```python
from build123d import *

# Parameters (mm, degrees)
BOSS_EXTRUDE1_DEPTH = 5
SKETCH2_R           = 4
CUT_EXTRUDE1_DEPTH  = 6


with BuildPart() as part:
    # Sketch1 → Boss-Extrude1 (new body)
    with BuildSketch(Plane(origin=(0, 0, 0), x_dir=(0, 0, -1), z_dir=(1, 0, 0))):
        with BuildLine():
            Line((-25, 10), (25, 10))
            ThreePointArc((25, 10), (35, 0), (25, -10))
            Line((25, -10), (-25, -10))
            ThreePointArc((-25, -10), (-35, 0), (-25, 10))
        make_face()
    extrude(amount=BOSS_EXTRUDE1_DEPTH)

    # Sketch2 → Cut-Extrude1 (cut, through all)
    with BuildSketch(Plane(origin=(5, 0, 0), x_dir=(0, 0, -1), z_dir=(1, 0, 0))):
        with Locations((-25, 0)):
            Circle(SKETCH2_R)
        with Locations((25, 0)):
            Circle(SKETCH2_R)
    extrude(amount=-CUT_EXTRUDE1_DEPTH, mode=Mode.SUBTRACT)


solid = part.part
```
Design review of the part built by this model. Coordinates are the model's own, in mm. Coordinates: 2 decimals unless noted, no trailing zeros. Loops run counter-clockwise (first coordinate to the right, second up) from the corner with the lowest first, then second, coordinate; pieces in that order, holes last.
Q1. We need section D-D on y = -3. State the section outline as (x, z) points, and give its area (3 significant figures).
Reported:
outline: (0, -34.54) - (5, -34.54) - (5, -27.65) - (0, -27.65) - close; (0, -22.35) - (5, -22.35) - (5, 22.35) - (0, 22.35) - close; (0, 27.65) - (5, 27.65) - (5, 34.54) - (0, 34.54) - close
area: 292 mm2
Q2. For pin 1 (9 mm diameter, centred on y = 0, z = -25, fed in from -X); pin 2 (3 mm diameter, centred on x = 1.5, y = -7.5, fed in from -Z); pin 3 (1 mm diameter, centred on x = 3, y = -7.5, fed in from +Z), all flat-tipped, find the tip position at first contact; note any pin that passes through.
Reported:
pin 1: stops at x = 0
pin 2: stops at z = -33
pin 3: stops at z = 32.14
Q3. To check wall thickness, follow line 1 (Y direction, x = 2.25, z = 25); line 2 (Z direction, x = 2.05, y = 2.5); line 3 (Z direction, x = 2.85, y = 2). State the ranges of each line that lie inside material, in increasing order.
Reported:
line 1: y = -10 to -4, 4 to 10
line 2: z = -34.68 to -28.12, -21.88 to 21.88, 28.12 to 34.68
line 3: z = -34.8 to -28.46, -21.54 to 21.54, 28.46 to 34.8
Q4. We need section A-A on y = 0. State the section outline as (x, z) points.
Reported:
outline: (0, -35) - (5, -35) - (5, -29) - (0, -29) - close; (0, -21) - (5, -21) - (5, 21) - (0, 21) - close; (0, 29) - (5, 29) - (5, 35) - (0, 35) - close
Q5. We need section B-B on z = -26. State the section outline as (x, y) points.
Reported:
outline: (0, -9.95) - (5, -9.95) - (5, -3.87) - (0, -3.87) - close; (0, 3.87) - (5, 3.87) - (5, 9.95) - (0, 9.95) - close
Q6. We need section C-C on x = 2.3. State the section outline as (y, z) points.
Reported:
outline: (-10, -25) arc R10 ccw to (10, -25) - (10, 25) arc R10 ccw to (-10, 25) - close; hole circle Ø8 at (0, -25); hole circle Ø8 at (0, 25)
